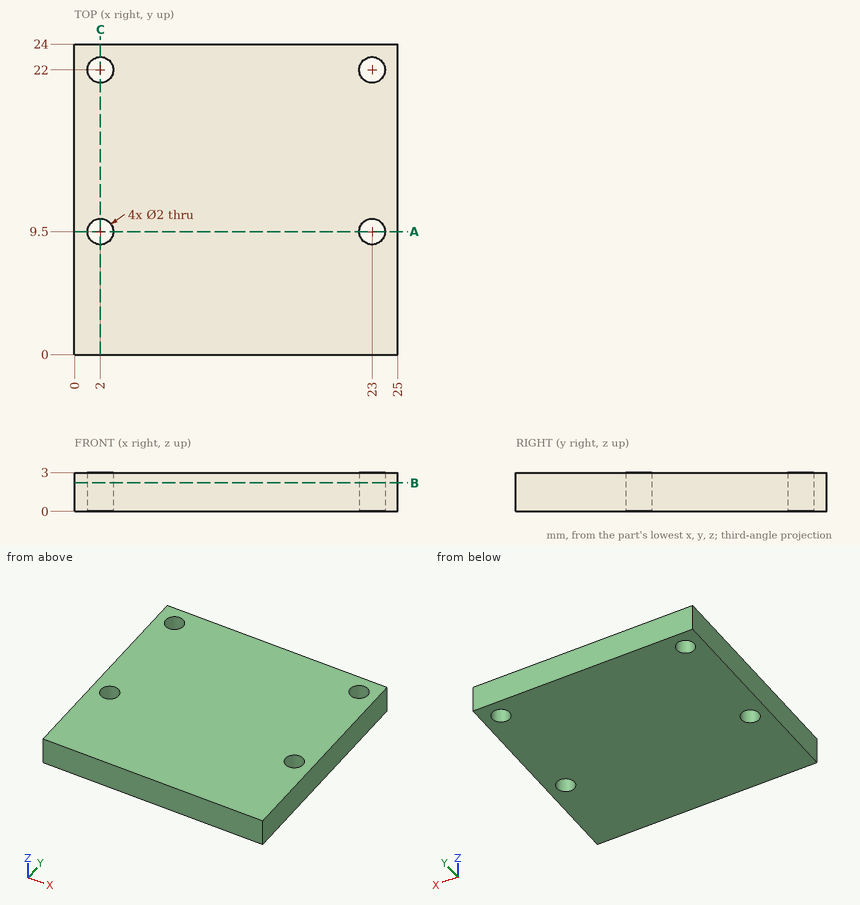
Study the drawing (mm; zero at the part's minimum x, y, z) and answer. Round coordinates to 2 decimals unless told otherwise and drop trailing zeros. Loops run counter-clockwise (first coordinate to the right, second up) from the corner with the lowest first, then second, coordinate; pieces in that order, holes last. Notation, with made-up numbers: (19.25, 72.5) - (74.25, 72.5) arc R18 cw to (74.25, 91.5) - close; hole circle Ø1 at (21.25, -14.5). An arc over 180 degrees is marked (long way). Use one line per item in the form item = value. Start each with the question number.
1. The part is cut by section B-B on z = 2.2. Determine the outline of the cut face in (x, y).
2. Consider line 1 (Y direction, x = 23, z = 1.9); line 2 (X direction, y = 10, z = 0.6); line 3 (Y direction, x = 22.5, z = 2.8). Determine where each line is inside the solid, lowest interval first. Write a range as [from, to].
3. The part is cut by section A-A on y = 9.5. Determine the outline of the cut face in (x, z).
4. The part is cut by section C-C on x = 2. Determine the outline of the cut face in (y, z), then the cut area to 3 significant figures.
Geometry check:
q1.outline = (0, 0) - (25, 0) - (25, 24) - (0, 24) - close; hole circle Ø2 at (2, 9.5); hole circle Ø2 at (2, 22); hole circle Ø2 at (23, 9.5); hole circle Ø2 at (23, 22)
q2.line_1 = [0, 8.5], [10.5, 21], [23, 24]
q2.line_2 = [0, 1.13], [2.87, 22.13], [23.87, 25]
q2.line_3 = [0, 8.63], [10.37, 21.13], [22.87, 24]
q3.outline = (0, 0) - (1, 0) - (1, 3) - (0, 3) - close; (3, 0) - (22, 0) - (22, 3) - (3, 3) - close; (24, 0) - (25, 0) - (25, 3) - (24, 3) - close
q4.outline = (0, 0) - (8.5, 0) - (8.5, 3) - (0, 3) - close; (10.5, 0) - (21, 0) - (21, 3) - (10.5, 3) - close; (23, 0) - (24, 0) - (24, 3) - (23, 3) - close
q4.area = 60.0 mm^2
